Geometry check sheet. Reference: the model listing, model coordinates, mm. A direction names the side the tool comes from. Coordinates: 2 decimals unless noted, no trailing zeros. Order: outer loops, then holes, each group sorted by start corner. A loop starts at its lowest first (then second) coordinate and runs counter-clockwise, first axis right, second up. Notation, with made-up numbers: M -30,-7.75 L -6,-7.75 A7 cw -6,1.25 Z; hole C 45,8.25 d8. An arc over 180 degrees is marked long. One line per item, written item: value. Start each with the question number.
1) Sectioned sample at A-A, the plane y = 0. Enter the section's corners in (x, z) (3 decimals).
2) Sectioned sample at C-C, the plane z = 0. Enter the section's corners in (x, y) (3 decimals), then the cut area to 3 significant figures.
3) Thickness scan on L1, parallel to Z at x = 4.5, y = 9; L2, parallel to Y at x = 3, z = -0.75; L3, parallel to Z at x = 3, y = 0 (3 decimals). Record the ranges inside material, lowest first. Write a range as from..to.
4) Sectioned sample at D-D, the plane x = 4.75. Enter the section's corners in (y, z) (3 decimals).
5) Draft check along Y on faces 4 (the cylindrical face through (3.195, 8.655, -1.341)), 5 (the flat face through (4.2, 8.4, -2.45)), 6 (the flat face through (3, 10.172, -1)). Enter one of: pulls with the +Y half, pulls with the -Y half, needs draft (parallel to the pull), parting line crosses it, or undercut.
6) Sectioned sample at B-B, the plane x = 3. Enter the section's corners in (y, z) (3 decimals).
7) Access from +Z, -Z, +X, -X, +Y, -Y to the whole of each face (thin tool, end or side, straight path). Record for faces 1 (the flat face through (3, 9, 2.45)), 2 (the flat face through (3, 5, -0.2)), 3 (the cylindrical face through (2.95, 4.47, -3.14)).
8) Go/stop test with flat-tipped pins: P1, Ø1.8, axis at x = 3.5, y = 8.5, coming from the +Z side; P2, Ø3, axis at x = 3, y = 6, coming from the +Z side; P3, Ø3.5, axis at x = 3, y = 7.17, coming from the -Z side. Record where each tip stops, or that it passes through.
Autodesk Inventor part; units mm, degrees
ref_plane "YZ Plane" through (0, 0, 0) normal (1, 0, 0) x (0, 1, 0)
ref_plane "XZ Plane" through (0, 0, 0) normal (0, 1, 0) x (-1, 0, 0)
ref_plane "XY Plane" through (0, 0, 0) normal (0, 0, 1) x (1, 0, 0)
sketch "Sketch1" plane through (0, 0, 0) normal (1, 0, 0) x (0, 1, 0)
  line L0 (0, 8.645) -> (0, -8.645)
  line L1 (-9.4444, 0) -> (13.4411, 0)
  circle A0 centre (0, 0) radius 6.175
  circle A1 centre (0, 0) radius 3.175
  line L2 (3.1687, -0.2) -> (6.1718, -0.2)
  line L3 (3.1687, 0.2) -> (6.1718, 0.2)
  line L4 (6.1718, 0.2) -> (10.1718, 0.2)
  line L5 (10.1718, 0.2) -> (10.1718, 2.45)
  line L6 (10.1718, 2.45) -> (5.6682, 2.45)
  line L7 (6.1718, -0.2) -> (10.1718, -0.2)
  line L8 (10.1718, -0.2) -> (10.1718, -2.45)
  line L9 (10.1718, -2.45) -> (5.6682, -2.45)
  dimension "d0" = 6.35
  dimension "d1" = 3
  dimension "d2" = 0.2
  dimension "d3" = 4
  dimension "d4" = 2.25
extrude "Extrusion1" add sketch "Sketch1" along normal blind 6 contours A0 L3 A1 L0 | L0 A1 L1 A0 | L6 L5 L4 A0 | L1 A1 L0 A0 | L0 A1 L2 A0 | A0 L7 L8 L9
sketch "Sketch2" plane through (0, 5.6682, -2.45) normal (0, 0, -1) x (-1, 0, 0)
  line L0 (0, 4.5036) -> (-6, 4.5036)
  circle A0 centre (-3, 1.5) radius 1.5
  circle A1 centre (-3, 1.5) radius 2.6 construction
  line L1 (0, 0) -> (-6, 0)
  point P0 (0, -5.6682)
  point P1 (-3, 4.5036)
  dimension "d8" = 3
  dimension "d24" = 5.2
extrude "Extrusion2" cut sketch "Sketch2" against normal up to surface (2.25 mm away)
sketch "Sketch4" plane through (0, 5.6682, 2.45) normal (0, 0, 1) x (1, 0, 0)
  circle A0 centre (3, 1.5) radius 1.5
  circle A1 centre (3, 1.5) radius 1.5
  circle A2 centre (3, 1.5) radius 1.425
  point P0 (0, -5.6682)
  point P1 (3, 0)
  dimension "d14" = 2.85
extrude "Extrusion4" cut sketch "Sketch4" against normal through all contours A2
fillet "Fillet2" radius 1 7 edges at (6, 10.1718, 1.325) (3, 5.6682, 2.45) (0, 10.1718, 1.325) (0, 10.1718, -1.325) (6, 10.1718, -1.325) (1.5, 5.6682, -2.45) (4.5, 5.6682, -2.45)
chamfer "Chamfer1" distance 0.5 angle 45 2 edges at (6, -3.175, 0) (0, -3.175, 0)
sketch "Sketch5" plane through (0, 6.2911, -2.45) normal (0, 0, -1) x (-1, 0, 0)
  arc A0 (-1.7831, 0) -> (-4.2169, 0) centre (-3, 0.8771) ccw
  circle A1 centre (-3, 0.8771) radius 2.7
  circle A2 centre (-3, 0.8771) radius 1.5
  point P0 (0, -6.2911)
  dimension "d25" = 5.4
extrude "Extrusion5" cut sketch "Sketch5" along normal through all contours A2 A0 | A1
chamfer "Chamfer2" distance 0.25 angle 45 16 edges at (6, -6.175, 0) (6, 9.1718, -1.325) (6, 7.7314, -2.45) (5.7071, 9.8789, -2.45) (3, 10.1718, -2.45) (0.2929, 9.8789, -2.45) (0, 7.7314, -2.45) (0, 9.1718, -1.325) (0, -6.175, 0) (0, 9.1718, 1.325) (0, 7.7314, 2.45) (0.2929, 9.8789, 2.45) (3, 10.1718, 2.45) (5.7071, 9.8789, 2.45) (6, 7.7314, 2.45) (6, 9.1718, 1.325)
sketch "Sketch3" plane through (0, 5.6682, 2.45) normal (0, 0, 1) x (1, 0, 0)
  circle A0 centre (2.5, 3.2518) radius 1.5
  circle A1 centre (2.5, 3.2518) radius 1.5
  line L0 (4.3187, 6.4018) -> (6.1373, 3.2518)
  line L1 (6.1373, 3.2518) -> (4.3187, 0.1018)
  line L2 (4.3187, 0.1018) -> (0.6813, 0.1018)
  line L3 (0.6813, 0.1018) -> (-1.1373, 3.2518)
  line L4 (-1.1373, 3.2518) -> (0.6813, 6.4018)
  line L5 (0.6813, 6.4018) -> (4.3187, 6.4018)
  point P0 (0, -5.6682)
  dimension "d11" = 6.3
properties part number "pipeClap"
Final values:
1. outline: M 0,-5.925 L 0.25,-6.175 L 5.75,-6.175 L 6,-5.925 L 6,-3.675 L 5.5,-3.175 L 0.5,-3.175 L 0,-3.675 Z; M 0,3.675 L 0.5,3.175 L 5.5,3.175 L 6,3.675 L 6,5.925 L 5.75,6.175 L 0.25,6.175 L 0,5.925 Z
2. outline: M 0,-5.925 L 0.25,-6.175 L 5.75,-6.175 L 6,-5.925 L 6,-3.675 L 5.5,-3.175 L 0.5,-3.175 L 0,-3.675 Z
2. area: 17.7 mm^2
3. L1: z = -2.45..-0.2, 0.2..2.45
3. L2: y = -6.13..-3.09, 3.09..5.67, 8.67..10.17
3. L3: z = -6.175..-3.175, 3.175..6.175
4. outline: M 3.169,-0.2 A3.175 cw long 3.169,0.2 L 10.172,0.2 L 10.172,2.2 L 9.922,2.45 L 6.291,2.45 A1 cw 5.414,2.969 A6.175 ccw long 5.112,-3.464 L 5.112,-2.45 L 9.922,-2.45 L 10.172,-2.2 L 10.172,-0.2 Z
5. face 4: undercut
5. face 5: needs draft
5. face 6: pulls with the +Y half
6. outline: M 3.169,-0.2 A3.175 cw long 3.169,0.2 L 5.743,0.2 L 5.743,2.613 A1 cw 5.414,2.969 A6.175 ccw long 4.468,-4.262 L 4.468,-2.45 L 5.668,-2.45 L 5.668,-0.2 Z; M 8.593,0.2 L 10.172,0.2 L 10.172,2.2 L 9.922,2.45 L 8.593,2.45 Z; M 8.668,-2.45 L 9.922,-2.45 L 10.172,-2.2 L 10.172,-0.2 L 8.668,-0.2 Z
7. face 1: +Z, +X, -X, +Y
7. face 2: +X, -X, +Y
7. face 3: -Z, +Y
8. P1: stops at z = 2.45
8. P2: stops at z = 4.23
8. P3: stops at z = -2.45
